Part model, mm, in its own coordinate system. Face numbers are marked on the shaded views. A direction names the side the tool comes from. Round coordinates to 2 decimals unless told otherwise and drop trailing zeros. Write each loop counter-clockwise with the first axis right and the second up, starting at its lowest first coordinate (ties: lowest second). Pieces come first, ordered by that corner, then holes. Notation, with made-up numbers: M 0.25,-3 L 18.25,-3 A11 cw 18.25,9 Z; hole C -13.75,14 d10. An arc over 180 degrees is marked long. Answer as a JSON object with one key per item and string values. Group by question number.
1. Drop flat-ended pins along their axis: pin 1 (8 mm diameter, centred on y = 19.5, z = -32, fed in from -X); pin 2 (3 mm diameter, centred on y = -46.5, z = -34, fed in from -X); pin 3 (18 mm diameter, centred on y = 0, z = 0, fed in from -X); pin 4 (2 mm diameter, centred on x = 43, y = 3.5, fed in from -Z). Give the stop position or say it passes through.
2. Which spindle directions (+Z, -Z, +X, -X, +Y, -Y) get a long thin tool onto all of the face, cutting with end or side? Do the marked faces 4, 5 and 6. Say none if no direction does.
3. Band-saw the part on D-D, the plane x = 9.5. Write the cut outline in (y, z).
4. Two-plate mould, pull along Z, no slides. Class the marked faces 1, 2 and 3: +Z half, -Z half, draft (parallel to the pull), parting line (faces both ways), or undercut.
5. Drill centre lines: line 1 (X direction, y = -0.5, z = 31.5); line 2 (Z direction, x = 24, y = -1); line 3 (X direction, y = -34, z = 34). Where is each one in solid material? Low to high. Write a range as from..to.
6. Band-saw the part on A-A, the plane z = 0. Write the cut outline in (x, y), plus the area to 3 significant figures.
7. Band-saw the part on C-C, the plane y = -32. Write the cut outline in (x, z).
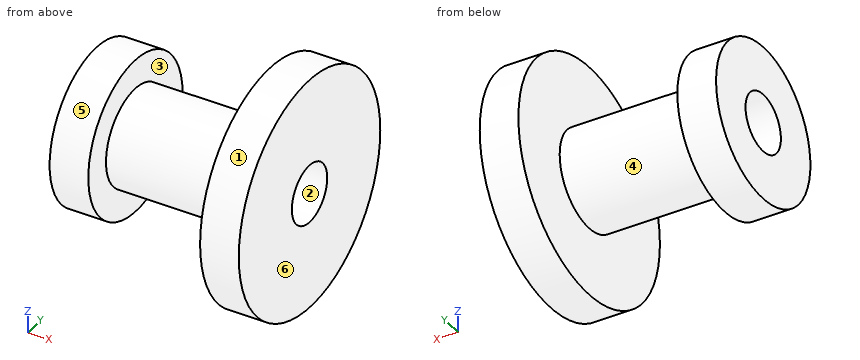
from build123d import *

# Parameters (mm, degrees)
SKETCH_3_R          = 15
CUT_EXTRUDE_1_DEPTH = 227


with BuildPart() as part:
    # 스케치2 → 회전1 (revolve)
    with BuildSketch(Plane.XY):
        Polygon((0, 0), (0, 40), (20, 40), (20, 25), (90, 25), (90, 60), (110, 60), (110, 0), align=None)
    revolve(axis=Axis((0, 0, 0), (1, 0, 0)))

    # 스케치3 → 컷-돌출1 (cut)
    with BuildSketch(Plane.ZY):
        Circle(SKETCH_3_R)
    extrude(amount=-CUT_EXTRUDE_1_DEPTH, mode=Mode.SUBTRACT)


solid = part.part
Worked answers:
{
 "1": {"pin 1": "stops at x = 0", "pin 2": "stops at x = 90", "pin 3": "passes through", "pin 4": "stops at z = -24.87"},
 "2": {"face 4": "none", "face 5": "-X", "face 6": "+Z, -Z, +X, +Y, -Y"},
 "3": {"outline": "C 0,0 d80; hole C 0,0 d30"},
 "4": {"face 1": "parting line", "face 2": "undercut", "face 3": "draft"},
 "5": {"line 1": "x = 0..20, 90..110", "line 2": "z = -24.98..-14.97, 14.97..24.98", "line 3": "x = 90..110"},
 "6": {"outline": "M 0,-40 L 20,-40 L 20,-25 L 90,-25 L 90,-60 L 110,-60 L 110,-15 L 0,-15 Z; M 0,15 L 110,15 L 110,60 L 90,60 L 90,25 L 20,25 L 20,40 L 0,40 Z", "area": "4,200 mm^2"},
 "7": {"outline": "M 0,-24 L 20,-24 L 20,24 L 0,24 Z; M 90,-50.75 L 110,-50.75 L 110,50.75 L 90,50.75 Z"}
}
